Design review of the part built by this model. Coordinates are the model's own, in mm. A direction names the side the tool comes from. Coordinates: 2 decimals unless noted, no trailing zeros. Order: outer loops, then holes, each group sorted by start corner. A loop starts at its lowest first (then second) coordinate and runs counter-clockwise, first axis right, second up. Notation, with made-up numbers: (42, 79) -> (94, 79) arc R9 cw to (94, 93) -> close; hole circle Ø4 at (27, 80.5). An arc over 180 degrees is marked (long way). Use a Markdown table: item, result. Add a question column.
Q1. Add section D-D (y = 0). State the section outline as (x, z) points, then the cut area to 3 significant figures.
Q2. Add section A-A (z = 0). State the section outline as (x, y) points.
Q3. Add section B-B (y = -32.5). State the section outline as (x, z) points.
Q4. Insertion check: pin 1 (10 mm diameter, centred on x = 38, y = 5.5, fed in from +Z); pin 2 (9 mm diameter, centred on x = 66, y = -4.5, fed in from -Z); pin 3 (8 mm diameter, centred on x = 29, z = -9.5, fed in from +Y). Each pin has a flat end and moves straight along its axis. Give the tip position at first contact, or say it passes through.
Q5. The part is to be moulded in two halves that separate along X. For faces 4 (the face through (115.14, 30.115, 0.751)), 5 (the face through (56, 0, 1.5)), 6 (the face through (104.86, -29.86, 0.14)), say which applies: pulls with the +X half, pulls with the -X half, needs draft (parallel to the pull), parting line crosses it, or undercut.
Q6. Add section C-C (x = 0). State the section outline as (y, z) points.
Q7. Wall thickness on probe 1 along Z at (x, y) = (115.5, -32.5); probe 2 along Y at (x, z) = (0, 3); probe 3 along Y at (x, z) = (119.5, 0): over which ranges is each line inside the solid? List them lowest first.
Q8. Machinability: for faces 1 (the face through (52.5, -14.93, 0.14)), 2 (the face through (95, 0, 6)), 3 (the face through (97, -3, -10)), which of the approach directions +Z, -Z, +X, -X, +Y, -Y give a long, thin tool a straight path to every point of the face, cutting with its end or side? Answer none if there is none.
from build123d import *

# Parameters (mm, degrees)
SKETCH001_R     = 15
SKETCH001_R_2   = 10
PAD_DEPTH       = 12.5
PAD001_DEPTH    = 10
PAD002_DEPTH    = 12.5
POCKET_DEPTH    = 337.344377
SKETCH006_R     = 2.5
POCKET001_DEPTH = 140.001


with BuildPart() as part:
    # Sketch001 → Pad (new body, symmetric)
    with BuildSketch(Plane.XY):
        Circle(SKETCH001_R)
        Circle(SKETCH001_R_2, mode=Mode.SUBTRACT)
    extrude(amount=PAD_DEPTH, both=True)

    # Sketch004 → Pad001 (join, symmetric)
    with BuildSketch(Plane.XY):
        with BuildLine():
            Line((125, 25), (125, 40))
            Line((125, 40), (115, 40))
            Line((115, 40), (95, 20))
            Line((95, 20), (11.18034, 10))
            ThreePointArc((11.18034, -10), (15, 0), (11.18034, 10))
            Line((11.18034, -10), (95, -20))
            Line((95, -20), (115, -40))
            Line((115, -40), (125, -40))
            Line((125, -40), (125, -25))
            ThreePointArc((125, 25), (100, 0), (125, -25))
        make_face()
    extrude(amount=PAD001_DEPTH, both=True)

    # Sketch003 → Pad002 (join, symmetric)
    with BuildSketch(Plane.XY):
        with BuildLine():
            ThreePointArc((125, 20), (105, 0), (125, -20))
            Line((125, -20), (125, -25))
            ThreePointArc((125, 25), (100, 0), (125, -25))
            Line((125, 25), (125, 20))
        make_face()
    extrude(amount=PAD002_DEPTH, both=True)

    # Sketch005 (on DatumPlane) → Pocket (cut, through all)
    with BuildSketch(Plane.XY.offset(1.5)):
        with BuildLine():
            ThreePointArc((25.737466, 8.715445), (18, 0), (25.737466, -8.715445))
            Line((25.737466, -8.715445), (78.140832, -14.967363))
            ThreePointArc((78.140832, -14.967363), (95, 0), (78.140832, 14.967363))
            Line((25.737466, 8.715445), (78.140832, 14.967363))
        make_face()
    pocket = extrude(amount=POCKET_DEPTH, mode=Mode.SUBTRACT)

    # Mirrored: Pocket across XY
    add(pocket.mirror(Plane.XY), mode=Mode.SUBTRACT)

    # Sketch006 (on DatumPlane) → Pocket001 (cut, through all)
    with BuildSketch(Plane(origin=(125, 0, 0), x_dir=(0, -1, 0), z_dir=(-1, 0, 0))):
        with Locations((-32.5, 0)):
            Circle(SKETCH006_R)
        with Locations((32.5, 0)):
            Circle(SKETCH006_R)
    extrude(amount=POCKET001_DEPTH, mode=Mode.SUBTRACT)


solid = part.part
Established:
| question | item | result |
|---|---|---|
| 1 | outline | (-15, -12.5) -> (-10, -12.5) -> (-10, 12.5) -> (-15, 12.5) -> close; (10, -12.5) -> (15, -12.5) -> (15, -10) -> (18, -10) -> (18, -1.5) -> (95, -1.5) -> (95, -10) -> (100, -10) -> (100, -12.5) -> (105, -12.5) -> (105, 12.5) -> (100, 12.5) -> (100, 10) -> (95, 10) -> (95, 1.5) -> (18, 1.5) -> (18, 10) -> (15, 10) -> (15, 12.5) -> (10, 12.5) -> close |
| 1 | area | 766 mm^2 |
| 2 | outline | (11.18, -10) -> (95, -20) -> (105, -30) -> (125, -30) -> (125, -20) arc R20 cw to (125, 20) -> (125, 30) -> (105, 30) -> (95, 20) -> (11.18, 10) arc R15 ccw (long way) to start; (110, -35) -> (115, -40) -> (125, -40) -> (125, -35) -> close; (110, 35) -> (125, 35) -> (125, 40) -> (115, 40) -> close; hole circle Ø20 at (0, 0) |
| 3 | outline | (107.5, -10) -> (125, -10) -> (125, -2.5) -> (107.5, -2.5) -> close; (107.5, 2.5) -> (125, 2.5) -> (125, 10) -> (107.5, 10) -> close |
| 4 | pin 1 | z = 10 |
| 4 | pin 2 | z = -1.5 |
| 4 | pin 3 | y = 12.6 |
| 5 | face 4 | needs draft |
| 5 | face 5 | undercut |
| 5 | face 6 | pulls with the -X half |
| 6 | outline | (-15, -12.5) -> (-10, -12.5) -> (-10, 12.5) -> (-15, 12.5) -> close; (10, -12.5) -> (15, -12.5) -> (15, 12.5) -> (10, 12.5) -> close |
| 7 | probe 1 | -10 to -2.5, 2.5 to 10 |
| 7 | probe 2 | -15 to -10, 10 to 15 |
| 7 | probe 3 | -40 to -35, -30 to -19.23, 19.23 to 30, 35 to 40 |
| 8 | face 1 | +Z, -Z, -Y |
| 8 | face 2 | +Z |
| 8 | face 3 | -Z |
